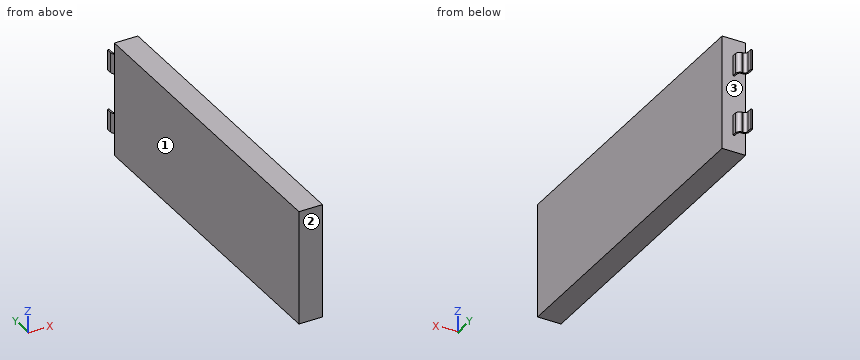
```python
from build123d import *

# Parameters (mm, degrees)
SKETCH_1_W      = 34
SKETCH_1_H      = 96
EXTRUDE_1_DEPTH = 7
EXTRUDE_2_DEPTH = 3


with BuildPart() as part:
    # 草图1 → 凸台-拉伸1 (new body)
    with BuildSketch(Plane(origin=(0, 0, 0), x_dir=(0, 0, -1), z_dir=(1, 0, 0))):
        Rectangle(SKETCH_1_W, SKETCH_1_H)
    extrude(amount=EXTRUDE_1_DEPTH)

    # 草图2 → 凸台-拉伸2 (add, symmetric)
    with BuildSketch(Plane.XY.offset(9)):
        with BuildLine():
            Line((3.25, 48), (3.25, 49.2))
            ThreePointArc((3.25, 49.2), (3.015685425, 49.765685425), (2.45, 50))
            Line((2.45, 50), (2.25, 50))
            ThreePointArc((2.25, 50), (1.245908371, 50.415908371), (0.83, 51.42))
            Line((0.83, 51.42), (0.83, 53))
            Line((0.83, 53), (1.33, 53))
            Line((1.33, 53), (1.33, 51.42))
            ThreePointArc((1.33, 51.42), (1.599461761, 50.769461761), (2.25, 50.5))
            Line((2.25, 50.5), (2.45, 50.5))
            ThreePointArc((2.45, 50.5), (3.369238816, 50.119238816), (3.75, 49.2))
            Line((3.75, 49.2), (3.75, 48))
            Line((3.75, 48), (3.25, 48))
        make_face()
    extrude_2 = extrude(amount=EXTRUDE_2_DEPTH, both=True)

    # 镜向1: 凸台-拉伸2 across plane
    add(extrude_2.mirror(Plane.XY))


solid = part.part
```
Source: CAD feature listing. Evaluate the final solid. Frame: model axes, mm. Face numbers are marked on the shaded views. Give positions to 0.01 mm unless a question says otherwise; leave off trailing zeros. Order: outer loops, then holes, each group sorted by start corner. A loop starts at its lowest first (then second) coordinate and runs counter-clockwise, first axis right, second up.
(1) Section query B-B (x = 5). Return the cut outline in (y, z).
(2) Material intervals for line 1 along Y through (x, z) = (3, 15.5), sorted ascending.
(3) Pull-direction query (Y, two-part tool) for the marked faces 1, 2 and 3; classes: +Y half, -Y half, draft (parallel to the pull), parting line (faces both ways), or undercut.
(4) Contact query for flat-ended pins moving along their axis: P1, Ø2, axis at x = 2, z = 3.5, coming from the +Y side; P2, Ø1, axis at y = 49, z = -9, coming from the -X side; P3, Ø0.5, axis at y = 52.5, z = -9, coming from the -X side. Output: stop coordinate, or through.
(5) Section query C-C (z = 0). Return the cut outline in (x, y).
(6) Section query A-A (z = 11). Return the cut outline in (x, y).
Outcome:
1. outline: (-48, -17) - (48, -17) - (48, 17) - (-48, 17) - close
2. line 1: y = -48 to 48
3. face 1: draft
3. face 2: -Y half
3. face 3: undercut
4. P1: stops at y = 48
4. P2: stops at x = 3.19
4. P3: stops at x = 0.83
5. outline: (0, -48) - (7, -48) - (7, 48) - (0, 48) - close
6. outline: (0, -48) - (7, -48) - (7, 48) - (3.75, 48) - (3.75, 49.2) arc R1.3 ccw to (2.45, 50.5) - (2.25, 50.5) arc R0.92 cw to (1.33, 51.42) - (1.33, 53) - (0.83, 53) - (0.83, 51.42) arc R1.42 ccw to (2.25, 50) - (2.45, 50) arc R0.8 cw to (3.25, 49.2) - (3.25, 48) - (0, 48) - close
